Check sheet for the drawn part. Datum: minimum x, y, z corner. Units: mm. A direction names the side the tool comes from. Coordinates: 2 decimals unless noted, no trailing zeros. Loops run counter-clockwise (first coordinate to the right, second up) from the corner with the lowest first, then second, coordinate; pieces in that order, holes last.
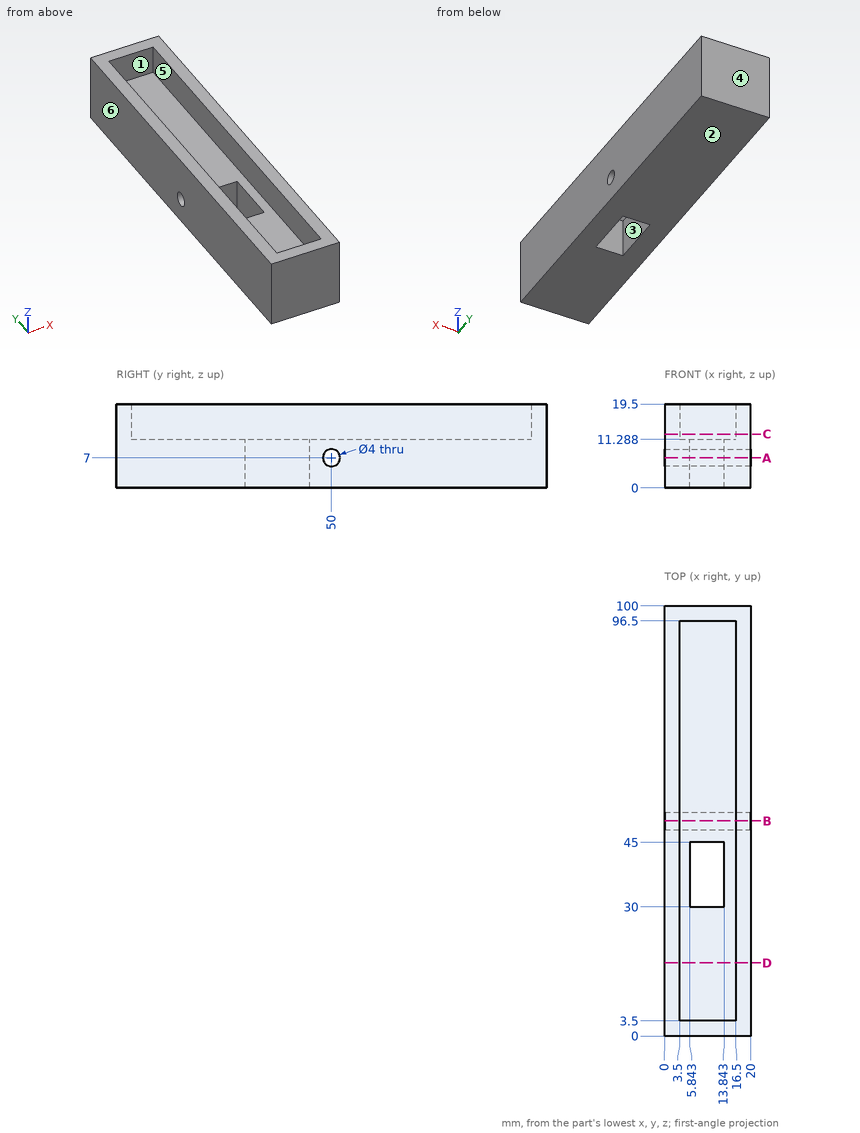
(1) Sectioned sample at B-B on y = 50. Record the cut outline in (x, z), and give its area (3 significant figures).
Findings:
outline: (0, 0) - (20, 0) - (20, 5) - (0, 5) - close; (0, 9) - (20, 9) - (20, 19.5) - (16.5, 19.5) - (16.5, 11.29) - (3.5, 11.29) - (3.5, 19.5) - (0, 19.5) - close
area: 203 mm2
(2) Scan lines: L1, parallel to Y at x = 13.5, z = 7; L2, parallel to Y at x = 9.25, z = 17; L3, parallel to X at y = 49, z = 15. Record each from-to range of solid material in increasing order.
Findings:
L1: y = 0 to 30, 45 to 48, 52 to 100
L2: y = 0 to 3.5, 96.5 to 100
L3: x = 0 to 3.5, 16.5 to 20
(3) Sectioned sample at A-A on z = 7. Record the cut outline in (x, y).
Findings:
outline: (0, 0) - (20, 0) - (20, 48) - (0, 48) - close; (0, 52) - (20, 52) - (20, 100) - (0, 100) - close; hole (5.84, 30) - (13.84, 30) - (13.84, 45) - (5.84, 45) - close
(4) Draft check along X on the marked faces 4, 5 and 6. Enter one of: +X half, -X half, draft (parallel to the pull), parting line (faces both ways), or undercut.
Findings:
face 4: draft
face 5: undercut
face 6: -X half
(5) Access from +Z, -Z, +X, -X, +Y, -Y to the whole of each face (thin tool, end or side, straight path). Record for the marked faces 1, 2 and 3.
Findings:
face 1: +Z
face 2: -Z, +X, -X, +Y, -Y
face 3: +Z, -Z
(6) Sectioned sample at D-D on y = 17. Record the cut outline in (x, z), and give its area (3 significant figures).
Findings:
outline: (0, 0) - (20, 0) - (20, 19.5) - (16.5, 19.5) - (16.5, 11.29) - (3.5, 11.29) - (3.5, 19.5) - (0, 19.5) - close
area: 283 mm2
(7) Sectioned sample at C-C on z = 12.5. Record the cut outline in (x, y).
Findings:
outline: (0, 0) - (20, 0) - (20, 100) - (0, 100) - close; hole (3.5, 3.5) - (16.5, 3.5) - (16.5, 96.5) - (3.5, 96.5) - close
(8) Gauge pin test, flat end, axial feed: pin 1 Ø4 at (x, y) = (7, 45) entering from +Z. Record the tip position at first contact, or that the pin passes through.
Findings:
pin 1: stops at z = 11.29
